Input: part model. Units: mm. Frame: model coordinates. A direction names the side the tool comes from. Give positions to 0.01 mm unless a question says otherwise; leave off trailing zeros. Write each loop counter-clockwise with the first axis right and the second up, starting at its lowest first coordinate (ties: lowest second). Pieces come first, ordered by that corner, then holes. Notation, with made-up numbers: (19.25, -27.75) - (65.25, -27.75) arc R29 cw to (65.25, -0.75) - close; hole circle Ø9 at (-22, 6.25). An arc over 180 degrees is marked (long way). Answer as CSV lines item,"result".
Autodesk Inventor part; units mm, degrees
ref_plane "YZ Plane" through (0, 0, 0) normal (1, 0, 0) x (0, 1, 0)
ref_plane "XZ Plane" through (0, 0, 0) normal (0, 1, 0) x (-1, 0, 0)
ref_plane "XY Plane" through (0, 0, 0) normal (0, 0, 1) x (1, 0, 0)
sketch "Sketch2" plane through (0, 0, 0) normal (0, 1, 0) x (-1, 0, 0)
  line L0 (0, 0) -> (0, -28)
  line L1 (0, -28) -> (22, -28)
  line L2 (22, -28) -> (22, 0)
  line L3 (22, 0) -> (0, 0)
  dimension "d0" = 28
  dimension "d1" = 22
extrude "Extrusion1" add sketch "Sketch2" along normal blind 4
sketch "Sketch3" plane through (0, 4, 0) normal (0, 1, 0) x (1, 0, 0)
  line L0 (0, 0) -> (0, 5)
  line L1 (0, 0) -> (0, 28)
  line L2 (0, 5) -> (-5, 5)
  circle A0 centre (-5, 5) radius 2.125
  dimension "d4" = 5
  dimension "d5" = 5
  dimension "d6" = 4.25
extrude "Extrusion2" cut sketch "Sketch3" against normal through all
pattern_linear "Rectangular Pattern1" count 2 spacing 18 along (0, 0, -1) count 3 spacing 6 along (-1, 0, 0) of "Extrusion2"
sketch "Sketch4" plane through (0, 4, 0) normal (0, 1, 0) x (1, 0, 0)
  point P0 (0, 0)
sketch "Sketch5" plane through (0, 0, 0) normal (1, 0, 0) x (0, 0, -1)
  line L0 (0, 4) -> (28, 4)
  line L1 (28, 4) -> (28, 0)
  line L2 (28, 0) -> (0, 0)
  line L3 (0, 0) -> (0, 4)
  line L4 (0, 4) -> (28, 4)
extrude "Extrusion3" add sketch "Sketch5" along normal blind 21.25
sketch "Sketch6" plane through (0, 0, 0) normal (0, -1, 0) x (1, 0, 0)
  line L0 (21.25, 0) -> (26.75, 0)
  line L1 (26.75, 0) -> (26.75, -28)
  line L2 (26.75, -28) -> (21.25, -28)
  line L3 (21.25, -28) -> (21.25, 0)
  point P0 (0, 0)
  dimension "d17" = 5.5
extrude "Extrusion4" add sketch "Sketch6" against normal blind 12.5
sketch "Sketch7" plane through (26.75, 0, 0) normal (1, 0, 0) x (0, 0, -1)
  line L0 (0, 4) -> (0, 12.5)
  line L1 (28, 12.5) -> (0, 12.5)
  line L2 (0, 12.5) -> (0, 5.25)
  line L3 (0, 5.25) -> (28, 5.25)
  line L4 (28, 5.25) -> (28, 12.5)
  point P0 (0, 0)
  dimension "d20" = 7.25
extrude "Extrusion5" add sketch "Sketch7" along normal blind 1.8
sketch "Sketch8" plane through (-22, 0, 0) normal (0, 0, 1) x (1, 0, 0)
  line L0 (50.55, 5.25) -> (43.25, 5.25)
  line L1 (43.25, 5.25) -> (43.25, 12.5)
  line L2 (43.25, 12.5) -> (50.55, 12.5)
  line L3 (50.55, 12.5) -> (50.55, 5.25)
  point P0 (22, 0)
extrude "Extrusion6" add sketch "Sketch8" along normal blind 5
fillet "Fillet1" radius 3 1 edges at (21.25, 8.875, 5)
fillet "Fillet2" radius 3 1 edges at (28.55, 8.875, 5)
sketch "Sketch9" plane through (-22, 0, -28) normal (0, 0, -1) x (-1, 0, 0)
  line L0 (-43.25, 12.5) -> (-50.55, 12.5)
  line L1 (-50.55, 12.5) -> (-50.55, 5.25)
  line L2 (-50.55, 5.25) -> (-43.25, 5.25)
  line L3 (-43.25, 5.25) -> (-43.25, 12.5)
  point P0 (-22, 0)
extrude "Extrusion7" add sketch "Sketch9" along normal blind 5
fillet "Fillet3" radius 3 1 edges at (28.55, 8.875, -33)
fillet "Fillet4" radius 3 1 edges at (21.25, 8.875, -33)
sketch "Sketch10" plane through (0, 12.5, 0) normal (0, 1, 0) x (1, 0, 0)
  line L0 (21.25, 28) -> (28.55, 28)
  line L1 (28.55, 30) -> (28.55, -2)
  line L2 (21.25, 28) -> (26.75, 28)
  line L3 (21.25, 0) -> (28.55, 0)
  line L4 (26.75, 0) -> (21.25, 0)
  line L5 (25.55, 33) -> (24.25, 33)
  line L6 (24.9, 33) -> (24.9, 28)
  line L7 (24.25, -5) -> (25.55, -5)
  line L8 (24.9, -5) -> (24.9, 0)
  circle A0 centre (24.9, 30.5) radius 1.5
  circle A1 centre (24.9, -2.5) radius 1.5
  point P0 (0, 0)
  dimension "d31" = 3
  dimension "d32" = 3
extrude "Extrusion8" cut sketch "Sketch10" against normal through all
properties part number "CartServoMount"
Item 1: Mould query, pull axis Z, two halves, no side actions, for faces 5 (the face through (-5.461, 2.028, -2.926)), 6 (the face through (27.65, 8.82, -32.14)), 7 (the face through (-11.461, 2.028, -20.926)), 8 (the face through (26.75, 3, -14)). Classes: +Z half, -Z half, draft (parallel to the pull), parting line (faces both ways), or undercut.
The answers:
face 5,"undercut"
face 6,"-Z half"
face 7,"undercut"
face 8,"draft"
Item 2: Ray query, line 1 (Z direction, x = -11, y = 3.25) (3 decimals); line 2 (X direction, y = 1.5, z = -23) (3 decimals); line 3 (Z direction, x = 24.9, y = 9.5). Return the intervals inside material, ascending. Write a range as from..to.
The answers:
line 1,"-28..-25.125, -20.875..-7.125, -2.875..0"
line 2,"-22..-19.125, -14.875..-13.125, -8.875..-7.125, -2.875..26.75"
line 3,"-33..-32, -29..1, 4..5"
Item 3: Reachability of faces 1 (the face through (2, 2, -28)), 2 (the face through (2, 2, 0)), 3 (the face through (-1, 4, -14)), 4 (the face through (-18.69, 2.03, -21.71)) from +Z, -Z, +X, -X, +Y, -Y: full face, straight path, thin tool, end or side. Return the list, or none.
The answers:
face 1,"-Z, +X, -X, -Y"
face 2,"+Z, +X, -X, -Y"
face 3,"+Z, -Z, -X, +Y"
face 4,"+Y, -Y"
Item 4: Cut plane A-A on x = 24.9. Return the cut outline in (y, z).
The answers:
outline,"(0, -28) - (5.25, -28) - (5.25, -29) - (12.5, -29) - (12.5, 1) - (5.25, 1) - (5.25, 0) - (0, 0) - close; (5.25, -33) - (12.5, -33) - (12.5, -32) - (5.25, -32) - close; (5.25, 4) - (12.5, 4) - (12.5, 5) - (5.25, 5) - close"
Item 5: Cut plane C-C on z = -5. Return the cut outline in (x, y) (3 decimals).
The answers:
outline,"(-22, 0) - (-19.125, 0) - (-19.125, 4) - (-22, 4) - close; (-14.875, 0) - (-13.125, 0) - (-13.125, 4) - (-14.875, 4) - close; (-8.875, 0) - (-7.125, 0) - (-7.125, 4) - (-8.875, 4) - close; (-2.875, 0) - (26.75, 0) - (26.75, 5.25) - (28.55, 5.25) - (28.55, 12.5) - (21.25, 12.5) - (21.25, 4) - (-2.875, 4) - close"
Item 6: Cut plane B-B on y = 6.25. Return the cut outline in (x, z), plus the area to 3 significant figures.
The answers:
outline,"(21.25, -30) arc R3 ccw to (24.25, -33) - (25.55, -33) arc R3 ccw to (28.55, -30) - (28.55, 2) arc R3 ccw to (25.55, 5) - (24.25, 5) arc R3 ccw to (21.25, 2) - close; hole circle Ø3 at (24.9, -30.5); hole circle Ø3 at (24.9, 2.5)"
area,"256 mm²"
Item 7: Cut plane D-D on y = 1.75. Return the cut outline in (x, z) (3 decimals), plus the area to 3 significant figures.
The answers:
outline,"(-22, -28) - (26.75, -28) - (26.75, 0) - (-22, 0) - close; hole circle Ø4.25 at (-17, -23); hole circle Ø4.25 at (-17, -5); hole circle Ø4.25 at (-11, -23); hole circle Ø4.25 at (-11, -5); hole circle Ø4.25 at (-5, -23); hole circle Ø4.25 at (-5, -5)"
area,"1,280 mm²"
Item 8: Contact query for flat-ended pins moving along their axis: pin 1 (5.5 mm diameter, centred on x = -11, z = -5, fed in from +Y); pin 2 (7 mm diameter, centred on y = 8, z = -8.5, fed in from -X); pin 3 (1.5 mm diameter, centred on y = 2.5, z = -18, fed in from +X). Output: stop coordinate, or through.
The answers:
pin 1,"y = 4"
pin 2,"x = 21.25"
pin 3,"x = 26.75"
